Source: three-view drawing plus pictorial views. Frame: mm from the lowest corner of the part. Round coordinates to 2 decimals unless told otherwise and drop trailing zeros. Loops run counter-clockwise (first coordinate to the right, second up) from the corner with the lowest first, then second, coordinate; pieces in that order, holes last. Notation, with made-up numbers: M -13,-11 L -6,-11 A13 cw -6,10 Z; hole C 0,25.5 d10. An arc over 180 degrees is marked long. Write each question's results on one line, items separated by ' | '.
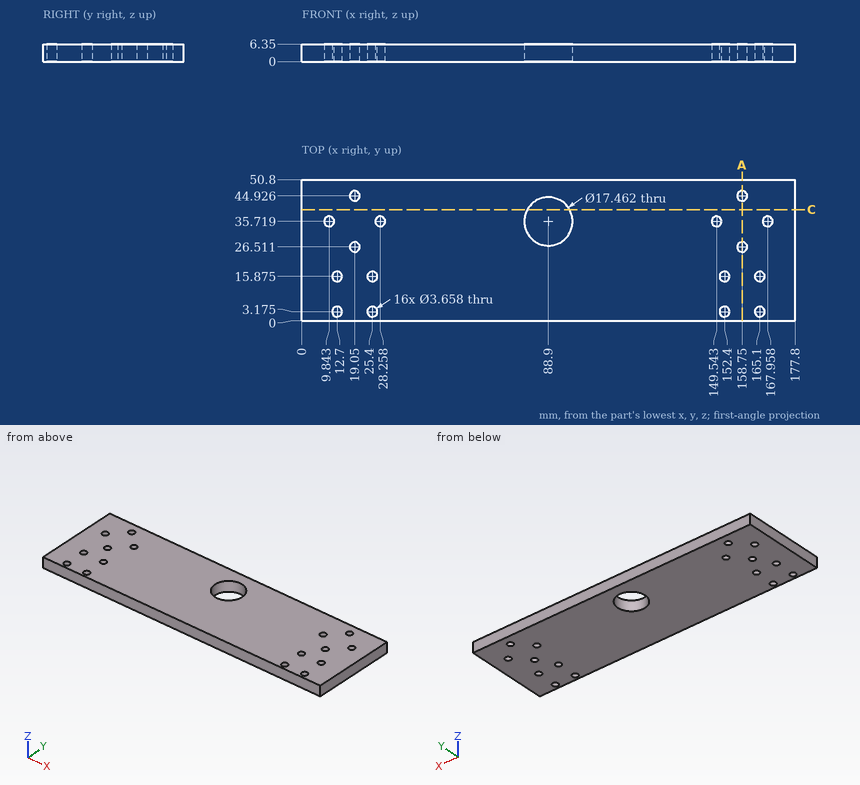
1. Ray query, probe 1 along Y at (x, z) = (152.4, 1.5); probe 2 along X at (y, z) = (26, 4) (1 decimal); probe 3 along X at (y, z) = (39, 3). Return the intervals inside material, ascending.
Answer key:
probe 1: y = 0 to 1.35, 5 to 14.05, 17.7 to 50.8 | probe 2: x = 0 to 17.3, 20.8 to 157, 160.5 to 177.8 | probe 3: x = 0 to 80.81, 96.99 to 177.8
2. Section A-A (x = 158.75). Count the separate pieces of the cut face and the enclosed holes in it, then the cut area to 3 significant figures.
Answer key:
separate pieces: 3 | enclosed holes: 0 | area: 276 mm²
3. Pin query (flat end, axial travel): P1, Ø2, axis at x = 158.75, y = 26.51, coming from the +Z side. Return the tip coordinate at first contact, or that it passes through.
Answer key:
P1: passes through
4. Section C-C (y = 40). Output: boundary loops of the cut face in (x, z), then the cut area to 3 significant figures.
Answer key:
outline: M 0,0 L 81.29,0 L 81.29,6.35 L 0,6.35 Z; M 96.51,0 L 177.8,0 L 177.8,6.35 L 96.51,6.35 Z | area: 1,030 mm²
